Source: three-view drawing plus pictorial views. Frame: mm from the lowest corner of the part. A direction names the side the tool comes from. Coordinates: 2 decimals unless noted, no trailing zeros. Loops run counter-clockwise (first coordinate to the right, second up) from the corner with the lowest first, then second, coordinate; pieces in that order, holes last. Notation, with made-up numbers: M -0.5,87.25 L 11.5,87.25 A12 cw 11.5,103.25 Z; hole C -32,51.25 d5. An arc over 180 degrees is marked long. Use a Markdown table: item, result. Add a question column.
1. Pin query (flat end, axial travel): pin 1 (2.5 mm diameter, centred on x = 8.89, y = 9.525, fed in from -Z); pin 2 (1.2 mm diameter, centred on x = 7, z = 3.5, fed in from +Y) (1 decimal); pin 3 (5 mm diameter, centred on x = 9.5, y = 7.5, fed in from +Z); pin 4 (5 mm diameter, centred on x = 9, y = 9.5, fed in from -Z). Return the tip coordinate at first contact, or that it passes through.
2. Set-up query: the marked faces 5, 6, 7, 8 and 9. Return all of +Z, -Z, +X, -X, +Y, -Y with unobstructed straight access to the full face (end or side cutting, diameter ignored); none if empty.
3. Section B-B on x = 5. Output: boundary loops of the cut face in (y, z) (1 decimal).
4. Section A-A on y = 8. State how many separate pieces and enclosed holes the cut face has.
5. Line query: L1, parallel to Z at x = 13.5, y = 8.25; L2, parallel to Y at x = 8.89, z = 3.2 (1 decimal); L3, parallel to X at y = 6.25, z = 7. Output: solid intervals per line, ascending. Write a range as [from, to].
6. Section D-D on y = 4.75. Output: boundary loops of the cut face in (x, z).
7. Draft query along Y for the marked faces 1, 2, 3 and 4. Return one class per face: +Y half, -Y half, draft (parallel to the pull), parting line (faces both ways), or undercut.
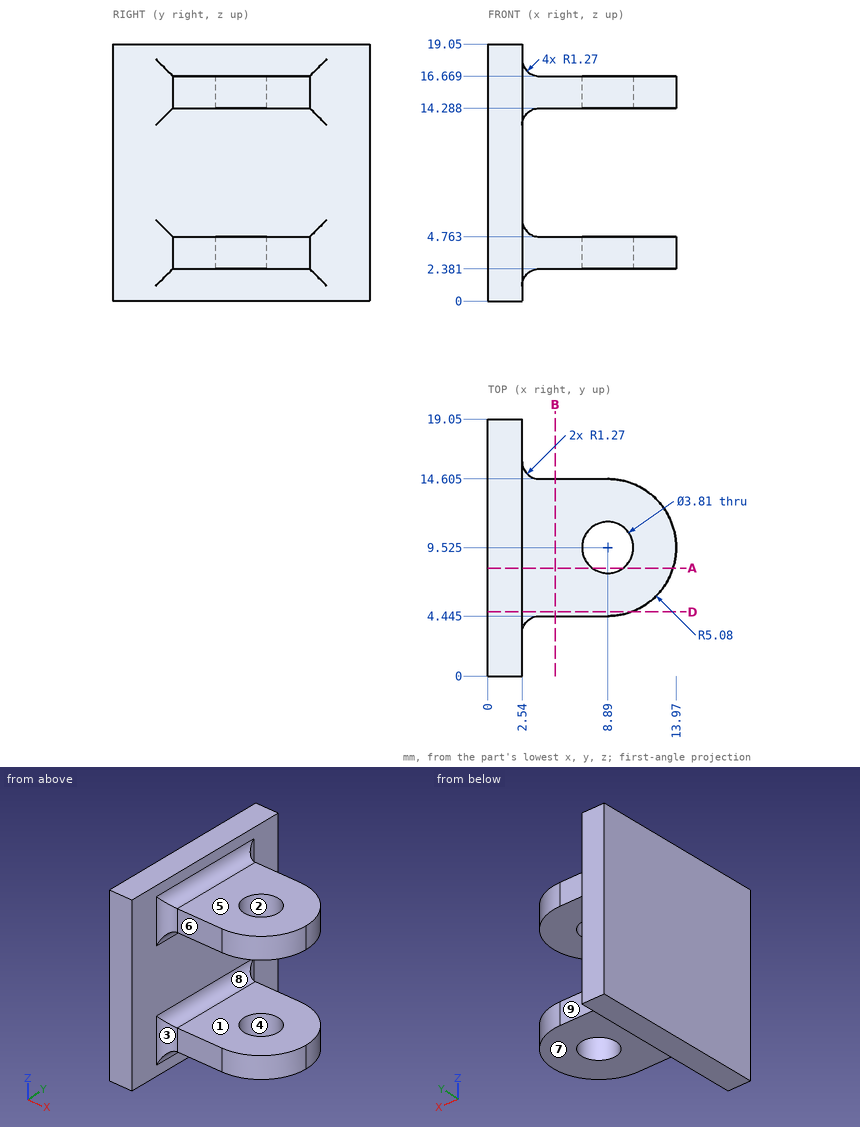
Answers below:
| question | item | result |
|---|---|---|
| 1 | pin 1 | passes through |
| 1 | pin 2 | stops at y = 14.6 |
| 1 | pin 3 | stops at z = 16.67 |
| 1 | pin 4 | stops at z = 2.38 |
| 2 | face 5 | +Z, +X, +Y, -Y |
| 2 | face 6 | +Z, -Z, +X, -Y |
| 2 | face 7 | -Z, +X, +Y, -Y |
| 2 | face 8 | +X, +Y, -Y |
| 2 | face 9 | +Z, -Z, +X, +Y |
| 3 | outline | M 4.4,2.4 L 14.6,2.4 L 14.6,4.8 L 4.4,4.8 Z; M 4.4,14.3 L 14.6,14.3 L 14.6,16.7 L 4.4,16.7 Z |
| 4 | separate pieces | 3 |
| 4 | enclosed holes | 0 |
| 5 | L1 | z = [2.38, 4.76], [14.29, 16.67] |
| 5 | L2 | y = [4.4, 7.6], [11.4, 14.6] |
| 5 | L3 | x = [0, 2.54] |
| 6 | outline | M 0,0 L 2.54,0 L 2.54,1.11 A1.27 cw 3.81,2.38 L 10.62,2.38 L 10.62,4.76 L 3.81,4.76 A1.27 cw 2.54,6.03 L 2.54,13.02 A1.27 cw 3.81,14.29 L 10.62,14.29 L 10.62,16.67 L 3.81,16.67 A1.27 cw 2.54,17.94 L 2.54,19.05 L 0,19.05 Z |
| 7 | face 1 | draft |
| 7 | face 2 | undercut |
| 7 | face 3 | -Y half |
| 7 | face 4 | undercut |
